The listing builds one solid part. Answer for the finished solid, in the listing's coordinates (mm). A direction names the side the tool comes from. Coordinates: 2 decimals unless noted, no trailing zeros. Order: outer loops, then holes, each group sorted by start corner. A loop starts at its lowest first (then second) coordinate and runs counter-clockwise, first axis right, second up. Notation, with made-up numbers: (51.25, -10.5) - (57.25, -10.5) arc R7 ccw to (57.25, -1.5) - close; hole circle Ø3 at (78, 55.25). An arc over 180 degrees is marked (long way). Use a Markdown table: item, result. Add a question column.
Item 1: Flat-ended cylindrical pins translate along their axes: P1, Ø3, axis at x = 5, z = -5, coming from the +Y side; P2, Ø1.5, axis at y = 12, z = -31.5, coming from the -X side; P3, Ø10, axis at x = 14.5, z = -29.5, coming from the +Y side. Find the tip coordinate at first contact, or state that the pin passes through.
Item 2: The part is cut by section C-C, the plane y = 36.5. Give the vertices of the cut face in (x, z).
Item 3: For faces 4 (the flat face through (0, 20, -20)), 5 (the flat face through (2, 21, -20)), determine the directions among +Z, -Z, +X, -X, +Y, -Y from which every point of the face is accessible in a straight line to the end or side of a thin tool.
Item 4: The part is cut by section D-D, the plane x = 15. Give the vertices of the cut face in (y, z).
Item 5: The part is cut by section A-A, the plane x = 35. Give the vertices of the cut face in (y, z).
Item 6: The mould has two halves that part along Z. Classify faces 1 (the flat face through (20, 20, 0)), 2 (the flat face through (20, 21, -38)), 3 (the flat face through (32, 40, -8)): released by +Z, released by -Z, zero draft, split by the parting line, or undercut.
Item 7: Find the intervals of material crossed by line 1 along Z through (x, y) = (35, 15); line 2 along X through (y, z) = (24.5, -35); line 3 along X through (y, z) = (11.5, -8), in increasing order.
Item 8: The part is cut by section B-B, the plane z = -35. Give the vertices of the cut face in (x, y).
Autodesk Inventor part; units mm, degrees
ref_plane "YZ Plane" through (0, 0, 0) normal (1, 0, 0) x (0, 1, 0)
ref_plane "XZ Plane" through (0, 0, 0) normal (0, 1, 0) x (-1, 0, 0)
ref_plane "XY Plane" through (0, 0, 0) normal (0, 0, 1) x (1, 0, 0)
sketch "cube_profile" plane through (0, 0, 0) normal (0, 1, 0) x (-1, 0, 0)
  line L0 (0, 0) -> (-40, 0)
  line L1 (-40, 0) -> (-40, -40)
  line L2 (-40, -40) -> (0, -40)
  line L3 (0, -40) -> (0, 0)
  dimension "d2" = 40
  dimension "d4" = 40
extrude "Extrusion1" add sketch "cube_profile" along normal blind 40
sketch "Sketch2" plane through (0, 40, 0) normal (0, 1, 0) x (1, 0, 0)
  line L0 (40, 40) -> (0, 40)
  line L1 (0, 40) -> (0, 0)
  circle A0 centre (5, 35) radius 2.5
  circle A1 centre (35, 35) radius 2.5
  circle A2 centre (5, 5) radius 2.5
  circle A3 centre (35, 5) radius 2.5
  dimension "d8" = 5
  dimension "d9" = 5
  dimension "d10" = 5
  dimension "d13" = 30
  dimension "d16" = 30
extrude "Extrusion2" cut sketch "Sketch2" against normal blind 50.325
shell "Shell1" thickness 2 removed faces 1 at (24.3762, 40, -24.4474)
sketch "Sketch3" plane through (0, 0, 0) normal (0, 0, 1) x (1, 0, 0)
  point P0 (0, 0)
properties part number "INTRO_CUBE"
Solution:
| question | item | result |
|---|---|---|
| 1 | P1 | passes through |
| 1 | P2 | stops at x = 0 |
| 1 | P3 | stops at y = 2 |
| 2 | outline | (0, -40) - (40, -40) - (40, 0) - (0, 0) - close; hole (2, -31.65) arc R4.5 cw to (8.35, -38) - (31.65, -38) arc R4.5 cw to (38, -31.65) - (38, -8.35) arc R4.5 cw to (31.65, -2) - (8.35, -2) arc R4.5 cw to (2, -8.35) - close; hole circle Ø5 at (5, -35); hole circle Ø5 at (5, -5); hole circle Ø5 at (35, -35); hole circle Ø5 at (35, -5) |
| 3 | face 4 | +Z, -Z, -X, +Y, -Y |
| 3 | face 5 | +Y |
| 4 | outline | (0, -40) - (40, -40) - (40, -38) - (2, -38) - (2, -2) - (40, -2) - (40, 0) - (0, 0) - close |
| 5 | outline | (0, -40) - (40, -40) - (40, -37.5) - (0, -37.5) - close; (0, -32.5) - (40, -32.5) - (40, -30.5) - (2, -30.5) - (2, -9.5) - (40, -9.5) - (40, -7.5) - (0, -7.5) - close; (0, -2.5) - (40, -2.5) - (40, 0) - (0, 0) - close |
| 6 | face 1 | released by +Z |
| 6 | face 2 | undercut |
| 6 | face 3 | zero draft |
| 7 | line 1 | z = -40 to -37.5, -32.5 to -30.5, -9.5 to -7.5, -2.5 to 0 |
| 7 | line 2 | x = 0 to 2.5, 7.5 to 9.5, 30.5 to 32.5, 37.5 to 40 |
| 7 | line 3 | x = 0 to 8.35, 31.65 to 40 |
| 8 | outline | (0, 0) - (2.5, 0) - (2.5, 40) - (0, 40) - close; (7.5, 0) - (32.5, 0) - (32.5, 40) - (30.5, 40) - (30.5, 2) - (9.5, 2) - (9.5, 40) - (7.5, 40) - close; (37.5, 0) - (40, 0) - (40, 40) - (37.5, 40) - close |
